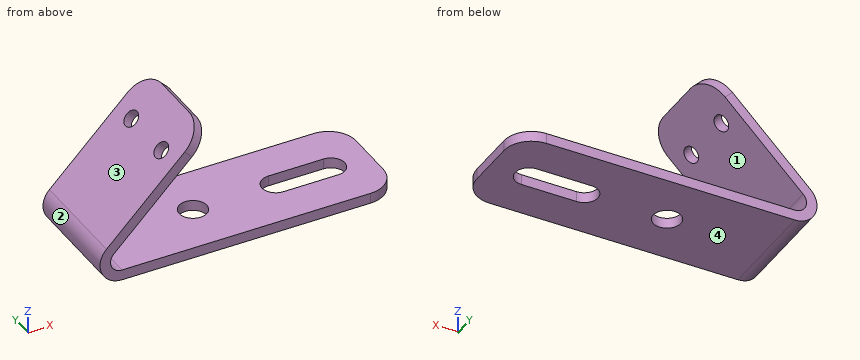
```python
from build123d import *

# Parameters (mm, degrees)
F1_DEPTH = 483.87
F2_R     = 38.1
F3_DEPTH = 48.26
F4_R     = 63.5
F5_DEPTH = 48.261
F6_R     = 127


with BuildPart() as f1:
    # F0 (on Front) → F1 (new body)
    with BuildSketch(Plane.XZ):
        with BuildLine():
            Line((-556.3015167441, 0), (713.6984832559, 0))
            Line((713.6984832559, 0), (713.6984832559, 48.26))
            Line((713.6984832559, 48.26), (-556.3015167441, 48.26))
            ThreePointArc((-556.3015167441, 48.26), (-605.5812510083, 81.1876657176), (-594.0185924526, 139.3170757085))
            Line((-594.0185924526, 139.3170757085), (-145.0057863992, 588.3298817619))
            Line((-145.0057863992, 588.3298817619), (-179.1307596592, 622.454855022))
            Line((-179.1307596592, 622.454855022), (-628.1435657127, 173.4420489685))
            ThreePointArc((-628.1435657127, 173.4420489685), (-650.1676772473, 62.7193632717), (-556.3015167441, 0))
        make_face()
    extrude(amount=F1_DEPTH)

    # F2 (on face) → F3 (cut, through all)
    with BuildSketch(Plane(origin=(-400.7928073406, 0, 400.7928073406), x_dir=(0, -1, 0), z_dir=(-0.7071067812, 0, 0.7071067812))):
        with Locations((114.3, 122.9774740944)):
            Circle(F2_R)
        with Locations((369.57, 122.9774740944)):
            Circle(F2_R)
    extrude(amount=-F3_DEPTH, mode=Mode.SUBTRACT)

    # F4 (on face) → F5 (cut, through all)
    with BuildSketch(Plane.XY.offset(48.26)):
        with BuildLine():
            Line((281.8984832559, -305.435), (535.8984832559, -305.435))
            ThreePointArc((535.8984832559, -305.435), (599.3984832559, -241.935), (535.8984832559, -178.435))
            Line((535.8984832559, -178.435), (281.8984832559, -178.435))
            ThreePointArc((281.8984832559, -178.435), (218.3984832559, -241.935), (281.8984832559, -305.435))
        make_face()
        with Locations((-99.1015167441, -241.935)):
            Circle(F4_R)
    extrude(amount=-F5_DEPTH, mode=Mode.SUBTRACT)

    # F6
    f6_edges = [f1.edges().sort_by_distance(p)[0] for p in [
        (713.698483, -483.87, 24.13),
        (713.698483, 0, 24.13),
        (-162.068273, 0, 605.392368),
        (-162.068273, -483.87, 605.392368),
    ]]
    fillet(f6_edges, radius=F6_R)


solid = f1.part
```
Work out the finished part from the listing and answer in its coordinate system (mm). Face numbers are marked on the shaded views. Give positions to 0.01 mm unless a question says otherwise; leave off trailing zeros. Loops run counter-clockwise (first coordinate to the right, second up) from the corner with the lowest first, then second, coordinate; pieces in that order, holes last. Notation, with made-up numbers: (66.5, -24.75) - (93.5, -24.75) arc R34 ccw to (93.5, 12.25) - close; hole circle Ø5 at (-34, -26). An arc over 180 degrees is marked (long way). One line per question, with ' | ' between items.
(1) The part is cut by section D-D (x = 22.5). Write down the section's boundary in (y, z).
Recorded:
outline: (-483.87, 0) - (0, 0) - (0, 48.26) - (-483.87, 48.26) - close
(2) The part is cut by section C-C (y = -59). Write down the section's boundary in (x, z).
Recorded:
outline: (-628.14, 173.44) arc R101.6 ccw to (-556.3, 0) - (693.96, 0) - (693.96, 48.26) - (-556.3, 48.26) arc R53.34 cw to (-594.02, 139.32) - (-158.96, 574.37) - (-193.09, 608.5) - close
(3) The part is cut by section A-A (y = -274). Write down the section's boundary in (x, z), then the cut area to 3 significant figures.
Recorded:
outline: (-628.14, 173.44) arc R101.6 ccw to (-556.3, 0) - (-153.91, 0) - (-153.91, 48.26) - (-556.3, 48.26) arc R53.34 cw to (-594.02, 139.32) - (-145.01, 588.33) - (-179.13, 622.45) - close; (-44.29, 0) - (227.09, 0) - (227.09, 48.26) - (-44.29, 48.26) - close; (590.71, 0) - (713.7, 0) - (713.7, 48.26) - (590.71, 48.26) - close | area: 77,900 mm²
(4) The part is cut by section B-B (y = -197). Write down the section's boundary in (x, z), then the cut area to 3 significant figures.
Recorded:
outline: (-628.14, 173.44) arc R101.6 ccw to (-556.3, 0) - (-143.97, 0) - (-143.97, 48.26) - (-556.3, 48.26) arc R53.34 cw to (-594.02, 139.32) - (-145.01, 588.33) - (-179.13, 622.45) - close; (-54.23, 0) - (237.03, 0) - (237.03, 48.26) - (-54.23, 48.26) - close; (580.77, 0) - (713.7, 0) - (713.7, 48.26) - (580.77, 48.26) - close | area: 79,800 mm²
(5) Each of these flat-tipped pins is pushed along its axis until it touches: pin 1 Ø4 at (x, y) = (379, -313.5) entering from -Z; pin 2 Ø1.5 at (y, z) = (-51.5, 214.5) entering from -X; pin 3 Ø1 at (y, z) = (-197.5, 499.5) entering from -X. Where does it stop, or does it pass through?
Recorded:
pin 1: stops at z = 0 | pin 2: stops at x = -587.84 | pin 3: stops at x = -302.59
(6) Straight lines are drawn through the part: probe 1 along Y at (x, z) = (-277.5, 457); probe 2 along Z at (x, y) = (-438.5, -215); probe 3 along Z at (x, y) = (614, -415.5). For each, find the intervals that lie inside material, in ascending order.
Recorded:
probe 1: y = -483.87 to -407.46, -331.68 to -152.19, -76.41 to 0 | probe 2: z = 0 to 48.26, 294.84 to 363.09 | probe 3: z = 0 to 48.26
(7) The mould has two halves that part along Z. Classify the marked faces 1, 2, 3 and 4: +Z half, -Z half, draft (parallel to the pull), parting line (faces both ways), or undercut.
Recorded:
face 1: undercut | face 2: parting line | face 3: +Z half | face 4: -Z half
